Read the model definition and answer for the solid it produces. Units are mm, in the model's axes. A direction names the side the tool comes from. Coordinates: 2 decimals unless noted, no trailing zeros. Order: outer loops, then holes, each group sorted by start corner. A loop starts at its lowest first (then second) coordinate and runs counter-clockwise, first axis right, second up.
```python
from build123d import *

# Parameters (mm, degrees)
SKETCH2_W           = 25
SKETCH2_H           = 25
SKETCH2_R           = 1.6
SKETCH2_W_2         = 0.5
SKETCH2_H_2         = 20
BOSS_EXTRUDE1_DEPTH = 8
SKETCH3_R           = 1.6
CUT_EXTRUDE1_DEPTH  = 37.249137921


with BuildPart() as part:
    # Sketch2 → Boss-Extrude1 (new body)
    with BuildSketch(Plane(origin=(0, 0, 0), x_dir=(1, 0, 0), z_dir=(0, 1, 0))):
        with Locations((12.5, 12.5)):
            Rectangle(SKETCH2_W, SKETCH2_H)
        with Locations(Location((12.5, 12.5, 0), (0, 0, 270))):
            Circle(SKETCH2_R, mode=Mode.SUBTRACT)
        with Locations((5, 12.5)):
            Rectangle(SKETCH2_W_2, SKETCH2_H_2, mode=Mode.SUBTRACT)
        with Locations((20, 12.5)):
            Rectangle(SKETCH2_W_2, SKETCH2_H_2, mode=Mode.SUBTRACT)
    extrude(amount=BOSS_EXTRUDE1_DEPTH)

    # Sketch3 → Cut-Extrude1 (cut, through all)
    with BuildSketch(Plane(origin=(25, 0, 0), x_dir=(0, 0, -1), z_dir=(1, 0, 0))):
        with Locations((7.5, 4)):
            Circle(SKETCH3_R)
        with Locations((17.5, 4)):
            Circle(SKETCH3_R)
    extrude(amount=-CUT_EXTRUDE1_DEPTH, mode=Mode.SUBTRACT)


solid = part.part
```
1) A cutting plane is placed at D-D, the plane z = -3.5. Determine the outline of the cut face in (x, y), and give its area (3 significant figures).
A:
outline: (0, 0) - (4.75, 0) - (4.75, 8) - (0, 8) - close; (5.25, 0) - (19.75, 0) - (19.75, 8) - (5.25, 8) - close; (20.25, 0) - (25, 0) - (25, 8) - (20.25, 8) - close
area: 192 mm2
2) Which of the six approach directions +Z, -Z, +X, -X, +Y, -Y give full straight-line access (tool end or side, diameter ignored) to faces 1 (the flat face through (12, 4, 0)), 2 (the flat face through (19.75, 4, -12))?
A:
face 1: +Z, +X, -X, +Y, -Y
face 2: +Y, -Y
3) A cutting plane is placed at C-C, the plane y = 7. Determine the outline of the cut face in (x, z), and give its area (3 significant figures).
A:
outline: (0, -25) - (25, -25) - (25, 0) - (0, 0) - close; hole (4.75, -22.5) - (5.25, -22.5) - (5.25, -2.5) - (4.75, -2.5) - close; hole circle Ø3.2 at (12.5, -12.5); hole (19.75, -22.5) - (20.25, -22.5) - (20.25, -2.5) - (19.75, -2.5) - close
area: 597 mm2
4) Determine the mould class of faces 3 (the cylindrical face through (22.66, 3.03, -6.23)), 4 (the flat face through (10, 0, -13)), 5 (the flat face through (5.25, 4, -12)) for opening direction Y: pulls with the +Y half, pulls with the -Y half, needs draft (parallel to the pull), parting line crosses it, or undercut.
A:
face 3: undercut
face 4: pulls with the -Y half
face 5: needs draft
5) A cutting plane is placed at B-B, the plane z = -17.5. Determine the outline of the cut face in (x, y).
A:
outline: (0, 0) - (4.75, 0) - (4.75, 2.4) - (0, 2.4) - close; (0, 5.6) - (4.75, 5.6) - (4.75, 8) - (0, 8) - close; (5.25, 0) - (19.75, 0) - (19.75, 2.4) - (5.25, 2.4) - close; (5.25, 5.6) - (19.75, 5.6) - (19.75, 8) - (5.25, 8) - close; (20.25, 0) - (25, 0) - (25, 2.4) - (20.25, 2.4) - close; (20.25, 5.6) - (25, 5.6) - (25, 8) - (20.25, 8) - close
6) A flat-ended cylindrical pin translates along its axis: pin 1 Ø2.5 at (y, z) = (4, -17.5) entering from +X. Find the tip coordinate at first contact, or state that the pin passes through.
A:
pin 1: passes through
7) Straight lines are drawn through the part: line 1 (X direction, y = 1, z = -5.75); line 2 (X direction, y = 5.5, z = -11.5); line 3 (Y direction, x = 14.5, z = -17.5). For each, find the intervals that lie inside material, in ascending order.
A:
line 1: x = 0 to 4.75, 5.25 to 19.75, 20.25 to 25
line 2: x = 0 to 4.75, 5.25 to 11.25, 13.75 to 19.75, 20.25 to 25
line 3: y = 0 to 2.4, 5.6 to 8
8) A cutting plane is placed at A-A, the plane x = 12.5. Determine the outline of the cut face in (y, z).
A:
outline: (0, -25) - (8, -25) - (8, -14.1) - (0, -14.1) - close; (0, -10.9) - (8, -10.9) - (8, 0) - (0, 0) - close; hole circle Ø3.2 at (4, -17.5); hole circle Ø3.2 at (4, -7.5)
